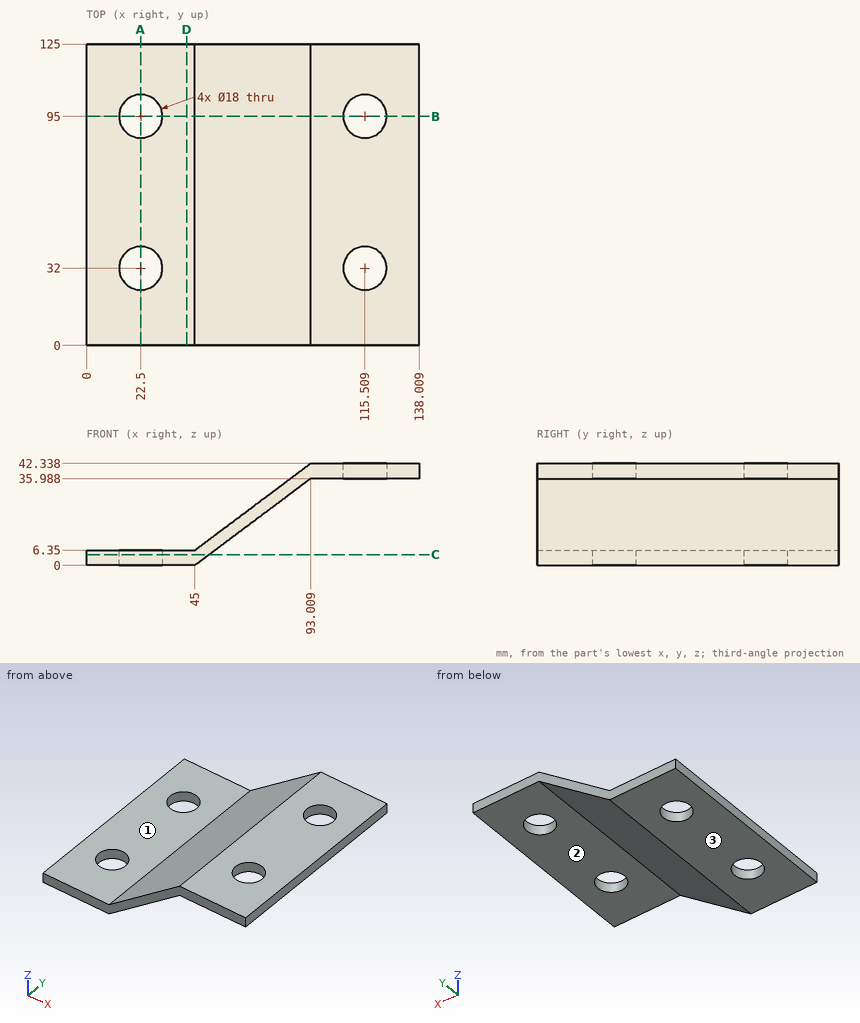
Print and shaded views of the part. All mm, measured from the part's lowest x, y and z. A direction names the side the tool comes from. Coordinates: 2 decimals unless noted, no trailing zeros. Write each loop counter-clockwise with the first axis right and the second up, starting at its lowest first coordinate (ties: lowest second). Pieces come first, ordered by that corner, then holes.
(1) 3-axis set-ups, long thin cutter, end or side, ignore diameter. For the marked faces 1, 2 and 3: which of +Z, -Z, +X, -X, +Y, -Y reach the whole face in a straight line?
(2) Cut at B-B, the plane y = 95. List the corners of the cut face in (x, z).
(3) Cut at A-A, the plane x = 22.5. List the corners of the cut face in (y, z), and give its area (3 significant figures).
(4) Cut at D-D, the plane x = 41.5. List the corners of the cut face in (y, z).
(5) Flat gauge pins, fed straight in: pin 1 (20.5 mm diameter, centred on x = 22.5, y = 95, fed in from +Z); pin 2 (1.5 mm diameter, centred on x = 45.5, y = 49, fed in from +Z); pin 3 (4 mm diameter, centred on x = 59, y = 44, fed in from +Z); pin 4 (12 mm diameter, centred on y = 70.5, z = 9.5, fed in from -X). Where does each tip first touch, or does it go through?
(6) Drill centre lines: probe 1 along Y at (x, z) = (22.5, 2.75); probe 2 along Z at (x, y) = (111, 112.5); probe 3 along Z at (x, y) = (7, 43). Where is each one in solid material? Low to high.
(7) Cut at C-C, the plane z = 4.5. List the corners of the cut face in (x, y), and give its area (3 significant figures).
Geometry says:
1. face 1: +Z, -X, +Y, -Y
1. face 2: -Z, +X, +Y, -Y
1. face 3: -Z, +X, -X, +Y, -Y
2. outline: (0, 0) - (13.5, 0) - (13.5, 6.35) - (0, 6.35) - close; (31.5, 0) - (45, 0) - (93.01, 35.99) - (106.51, 35.99) - (106.51, 42.34) - (93.01, 42.34) - (45, 6.35) - (31.5, 6.35) - close; (124.51, 35.99) - (138.01, 35.99) - (138.01, 42.34) - (124.51, 42.34) - close
3. outline: (0, 0) - (23, 0) - (23, 6.35) - (0, 6.35) - close; (41, 0) - (86, 0) - (86, 6.35) - (41, 6.35) - close; (104, 0) - (125, 0) - (125, 6.35) - (104, 6.35) - close
3. area: 565 mm2
4. outline: (0, 0) - (125, 0) - (125, 6.35) - (0, 6.35) - close
5. pin 1: stops at z = 6.35
5. pin 2: stops at z = 7.29
5. pin 3: stops at z = 18.34
5. pin 4: stops at x = 0
6. probe 1: y = 0 to 23, 41 to 86, 104 to 125
6. probe 2: z = 35.99 to 42.34
6. probe 3: z = 0 to 6.35
7. outline: (0, 0) - (51, 0) - (51, 125) - (0, 125) - close; hole circle Ø18 at (22.5, 32); hole circle Ø18 at (22.5, 95)
7. area: 5,870 mm2
